```python
from build123d import *

# Parameters (mm, degrees)
SKETCH1_R               = 2.75
BOSS_EXTRUDE1_DEPTH     = 4
FILLET1_R               = 5
BOSS_EXTRUDE3_DEPTH     = 9.6
BOSS_EXTRUDE4_DEPTH     = 10
BOSS_EXTRUDE5_DEPTH     = 4
BOSS_EXTRUDE6_START     = -12
BOSS_EXTRUDE6_DEPTH     = 12
CUT_EXTRUDE1_START      = -10
CUT_EXTRUDE1_DEPTH      = 10
BOSS_EXTRUDE7_DEPTH     = 4
BOSS_EXTRUDE8_START     = -7.6
BOSS_EXTRUDE8_DEPTH     = 7.6
BOSS_EXTRUDE9_START     = 2
BOSS_EXTRUDE9_DEPTH     = 2
FILLET2_R               = 7
SKETCH15_W              = 8.45
SKETCH15_H              = 80
CUT_EXTRUDE2_DEPTH      = 14
FILLET3_R               = 2
CUT_EXTRUDE4_DEPTH      = 132.997651535
CUT_EXTRUDE4_DEPTH_BACK = 132.997651535
SKETCH17_R              = 2.75


with BuildPart() as part:
    # Sketch1 → Boss-Extrude1 (new body)
    with BuildSketch(Plane.XY):
        Polygon((-62.15, 75), (-69.55, 75), (-69.55, 65.75), (-62.15, 65.75), (-62.15, 64.25), (-69.55, 64.25), (-69.55, 55), (-62.15, 55), (-62.15, 11.5), (-41.85, 11.5), (-41.85, 55), (-34.45, 55), (-34.45, 64.25), (-41.85, 64.25), (-41.85, 65.75), (-34.45, 65.75), (-34.45, 75), (-41.85, 75), (-41.85, 118.5), (-62.15, 118.5), align=None)
        with Locations((-52, 111.75)):
            Circle(SKETCH1_R, mode=Mode.SUBTRACT)
        with Locations((-52, 18.25)):
            Circle(SKETCH1_R, mode=Mode.SUBTRACT)
    extrude(amount=BOSS_EXTRUDE1_DEPTH)

    # Fillet1
    fillet1_edges = [part.edges().sort_by_distance(p)[0] for p in [
        (-62.15, 118.5, 2),
        (-41.85, 118.5, 2),
        (-41.85, 11.5, 2),
        (-62.15, 11.5, 2),
    ]]
    fillet(fillet1_edges, radius=FILLET1_R)



with BuildPart() as body_2:
    # Sketch3 → Boss-Extrude3 (new body)
    with BuildSketch(Plane(origin=(-34.45, 0, 0), x_dir=(0, 0, -1), z_dir=(1, 0, 0))):
        with BuildLine():
            Line((-12.8, 65), (-4, 65))
            Line((-4, 65), (-4, 65.75))
            Line((-4, 65.75), (-4, 75))
            Line((-4, 75), (-4, 98.135455405))
            ThreePointArc((-4, 98.135455405), (-8.435930345, 85.488200598), (-19.8, 78.382677882))
            Line((-19.8, 78.382677882), (-19.8, 75.382677882))
            ThreePointArc((-19.8, 75.382677882), (-14.713450587, 71.260990337), (-12.8, 65))
        make_face()
        with BuildLine():
            Line((-4, 31.864544449), (-4, 65))
            Line((-4, 65), (-12.8, 65))
            ThreePointArc((-12.8, 65), (-14.713450587, 58.739009663), (-19.8, 54.617322118))
            Line((-19.8, 54.617322118), (-19.8, 51.617322118))
            ThreePointArc((-19.8, 51.617322118), (-8.435930299, 44.511799345), (-4, 31.864544449))
        make_face()
    extrude(amount=BOSS_EXTRUDE3_DEPTH)


with BuildPart() as part_1:
    add(part.part)

    add(body_2.part)  # Boss-Extrude4 merges body 2
    # Sketch5 → Boss-Extrude4 (add)
    with BuildSketch(Plane.ZY.offset(34.45)):
        with BuildLine():
            Line((4, 98.135455551), (4, 31.864544449))
            ThreePointArc((4, 31.864544449), (8.435930299, 44.511799345), (19.8, 51.617322118))
            Line((19.8, 51.617322118), (19.8, 54.617322118))
            ThreePointArc((19.8, 54.617322118), (12.8, 65), (19.8, 75.382677882))
            Line((19.8, 75.382677882), (19.8, 78.382677882))
            ThreePointArc((19.8, 78.382677882), (8.435930299, 85.488200655), (4, 98.135455551))
        make_face()
    extrude(amount=BOSS_EXTRUDE4_DEPTH)

    # Sketch6 → Boss-Extrude5 (add)
    with BuildSketch(Plane(origin=(0, 0, 4), x_dir=(-1, 0, 0), z_dir=(0, 0, -1))):
        Polygon((24.85, 31.864544449), (41.85, 31.864544449), (41.85, 55), (34.45, 55), (34.45, 64.25), (41.85, 64.25), (41.85, 65.75), (34.45, 65.75), (34.45, 75), (41.85, 75), (41.85, 98.135455551), (24.85, 98.135455551), align=None)
    extrude(amount=BOSS_EXTRUDE5_DEPTH)

    # Sketch9 → Boss-Extrude6 (add)
    with BuildSketch(Plane.ZY.offset(44.45).offset(BOSS_EXTRUDE6_START)):
        with BuildLine():
            Line((4, 31.864544449), (5, 31.864544449))
            ThreePointArc((5, 31.864544449), (9.468774813, 44.195523989), (20.8, 50.800547872))
            Line((20.8, 50.800547872), (20.8, 55.31495999))
            ThreePointArc((20.8, 55.31495999), (20.485627959, 55.424552796), (20.175, 55.544346929))
            ThreePointArc((20.175, 55.544346929), (13.8, 65), (20.175, 74.455653071))
            ThreePointArc((20.175, 74.455653071), (20.485627959, 74.575447204), (20.8, 74.68504001))
            Line((20.8, 74.68504001), (20.8, 79.199452128))
            ThreePointArc((20.8, 79.199452128), (9.468774813, 85.804476011), (5, 98.135455551))
            Line((5, 98.135455551), (4, 98.135455551))
            ThreePointArc((4, 98.135455551), (8.435930299, 85.488200655), (19.8, 78.382677882))
            Line((19.8, 78.382677882), (19.8, 75.382677882))
            ThreePointArc((19.8, 75.382677882), (12.8, 65), (19.8, 54.617322118))
            Line((19.8, 54.617322118), (19.8, 51.617322118))
            ThreePointArc((19.8, 51.617322118), (8.435930299, 44.511799345), (4, 31.864544449))
        make_face()
    extrude(amount=BOSS_EXTRUDE6_DEPTH)

    # Sketch10 → Cut-Extrude1 (cut)
    with BuildSketch(Plane.ZY.offset(44.45).offset(CUT_EXTRUDE1_START)):
        with BuildLine():
            Line((4, 98.135455551), (4, 31.864544449))
            Line((4, 31.864544449), (5, 31.864544449))
            ThreePointArc((5, 31.864544449), (9.468774813, 44.195523989), (20.8, 50.800547872))
            Line((20.8, 50.800547872), (20.8, 55.31495999))
            ThreePointArc((20.8, 55.31495999), (13.8, 65), (20.8, 74.68504001))
            Line((20.8, 74.68504001), (20.8, 79.199452128))
            ThreePointArc((20.8, 79.199452128), (9.468774813, 85.804476011), (5, 98.135455551))
            Line((5, 98.135455551), (4, 98.135455551))
        make_face()
    extrude(amount=CUT_EXTRUDE1_DEPTH, mode=Mode.SUBTRACT)

    # Sketch12 → Boss-Extrude7 (add)
    with BuildSketch(Plane.XY.offset(4)):
        Polygon((-79.15, 31.864544449), (-62.15, 31.864544449), (-62.15, 55), (-69.55, 55), (-69.55, 64.25), (-62.15, 64.25), (-62.15, 65.75), (-69.55, 65.75), (-69.55, 75), (-62.15, 75), (-62.15, 98.135455551), (-79.15, 98.135455551), align=None)
    extrude(amount=-BOSS_EXTRUDE7_DEPTH)

    # Sketch13 → Boss-Extrude8 (add)
    with BuildSketch(Plane.ZY.offset(79.15).offset(BOSS_EXTRUDE8_START)):
        with BuildLine():
            Line((19.8, 75.382677882), (19.8, 78.382677882))
            ThreePointArc((19.8, 78.382677882), (8.435930299, 85.488200655), (4, 98.135455551))
            Line((4, 98.135455551), (0, 98.135455551))
            Line((0, 98.135455551), (0, 31.864544449))
            Line((0, 31.864544449), (4, 31.864544449))
            ThreePointArc((4, 31.864544449), (8.435930299, 44.511799345), (19.8, 51.617322118))
            Line((19.8, 51.617322118), (19.8, 54.617322118))
            ThreePointArc((19.8, 54.617322118), (12.8, 65), (19.8, 75.382677882))
        make_face()
    extrude(amount=BOSS_EXTRUDE8_DEPTH)

    # Sketch14 → Boss-Extrude9 (add)
    with BuildSketch(Plane(origin=(-71.55, 0, 0), x_dir=(0, 0, -1), z_dir=(1, 0, 0)).offset(BOSS_EXTRUDE9_START)):
        with BuildLine():
            Line((-4, 98.135455551), (-5, 98.135455551))
            ThreePointArc((-5, 98.135455551), (-9.468774813, 85.804476011), (-20.8, 79.199452128))
            Line((-20.8, 79.199452128), (-20.8, 74.68504001))
            ThreePointArc((-20.8, 74.68504001), (-13.8, 65), (-20.8, 55.31495999))
            Line((-20.8, 55.31495999), (-20.8, 50.800547872))
            ThreePointArc((-20.8, 50.800547872), (-9.468774813, 44.195523989), (-5, 31.864544449))
            Line((-5, 31.864544449), (-4, 31.864544449))
            Line((-4, 31.864544449), (-4, 98.135455551))
        make_face()
    extrude(amount=-BOSS_EXTRUDE9_DEPTH)

    # Fillet2
    fillet2_edges = [part_1.edges().sort_by_distance(p)[0] for p in [
        (-24.85, 98.135455551, 2),
        (-24.85, 31.864544449, 2),
        (-41.85, 31.864544449, 2),
        (-41.85, 98.135455551, 2),
        (-79.15, 31.864544449, 2),
        (-79.15, 98.135455551, 2),
        (-62.15, 98.135455551, 2),
        (-62.15, 31.864544449, 2),
    ]]
    fillet(fillet2_edges, radius=FILLET2_R)

    # Sketch15 → Cut-Extrude2 (cut)
    with BuildSketch(Plane(origin=(0, 0, 0), x_dir=(-1, 0, 0), z_dir=(0, 0, -1))):
        with Locations((52, 65)):
            Rectangle(SKETCH15_W, SKETCH15_H)
    extrude(amount=-CUT_EXTRUDE2_DEPTH, mode=Mode.SUBTRACT)

    # Fillet3
    fillet3_edges = [part_1.edges().sort_by_distance(p)[0] for p in [
        (-28.65, 75.382677882, 19.8),
        (-28.65, 78.382677882, 19.8),
        (-28.65, 54.617322118, 19.8),
        (-28.65, 51.617322118, 19.8),
        (-33.45, 50.800547872, 20.8),
        (-33.45, 79.199452128, 20.8),
        (-33.45, 74.68504001, 20.8),
        (-33.45, 55.31495999, 20.8),
        (-75.35, 78.382677882, 19.8),
        (-75.35, 75.382677882, 19.8),
        (-75.35, 54.617322118, 19.8),
        (-75.35, 51.617322118, 19.8),
        (-70.55, 79.199452128, 20.8),
        (-70.55, 74.68504001, 20.8),
        (-70.55, 55.31495999, 20.8),
        (-70.55, 50.800547872, 20.8),
    ]]
    fillet(fillet3_edges, radius=FILLET3_R)

    # Sketch17 → Cut-Extrude4 (cut, two sides: drawn at the far end of the back side and taken through both)
    with BuildSketch(Plane(origin=(-24.85, 0, 0), x_dir=(0, 0, -1), z_dir=(1, 0, 0)).offset(-CUT_EXTRUDE4_DEPTH_BACK)):
        with Locations((-8.8, 75)):
            Circle(SKETCH17_R)
        with Locations((-8.8, 55)):
            Circle(SKETCH17_R)
    extrude(amount=CUT_EXTRUDE4_DEPTH + CUT_EXTRUDE4_DEPTH_BACK, mode=Mode.SUBTRACT)


solid = part_1.part
```
Model file for the job. Use its own axes, mm. A direction names the side the tool comes from. Coordinates: 2 decimals unless noted, no trailing zeros. Write each loop counter-clockwise with the first axis right and the second up, starting at its lowest first coordinate (ties: lowest second). Pieces come first, ordered by that corner, then holes. Notation, with made-up numbers: (28.5, 5.5) - (32.5, 5.5) arc R28 ccw to (32.5, 35.5) - close; hole circle Ø2 at (32, -11.5). An arc over 180 degrees is marked (long way). Use a Markdown table: item, result. Add a question column.
Item 1: Drop flat-ended pins along their axis: pin 1 (3.5 mm diameter, centred on x = -70.5, z = 2.5, fed in from -Y); pin 2 (3.5 mm diameter, centred on x = -70, z = 2, fed in from +Y); pin 3 (7 mm diameter, centred on x = -52, y = 18.25, fed in from +Z); pin 4 (3.5 mm diameter, centred on y = 75, z = 8.8, fed in from -X). Give the stop position or say it passes through.
Item 2: 3-axis set-ups, long thin cutter, end or side, ignore diameter. For faces 4 (the face through (-28.703, 86.216, 7.88)), 5 (the face through (-44, 66, 4)), 6 (the face through (-75.297, 43.784, 7.88)): which of +Z, -Z, +X, -X, +Y, -Y reach the whole face in a straight line?
Item 3: Band-saw the part on C-C, the plane x = -52. Write the cut outline in (y, z), and give its area (3 significant figures).
Item 4: Band-saw the part on A-A, the plane z = 2. Give the number of separate pieces and of enclosed holes in the cut face, and give its area (3 significant figures).
Item 5: Band-saw the part on B-B, the plane y = 111.75. Write the cut outline in (x, z), and give its area (3 significant figures).
Item 6: Drill centre lines: line 1 along X through (y, z) = (54, 2.25) (3 decimals); line 2 along X through (y, z) = (66.5, 7.5); line 3 along Y through (x, z) = (-53, 2). Where is each one in solid material? Low to high.
Item 7: Two-plate mould, pull along X, no slides. Class faces 1 (the face through (-56.225, 64, 2)), 2 (the face through (-62.15, 21, 2)), 3 (the face through (-75.3, 64.8, 12.8)): pulls with the +X half, pulls with the -X half, needs draft (parallel to the pull), parting line crosses it, or undercut.
A:
| question | item | result |
|---|---|---|
| 1 | pin 1 | stops at y = 31.85 |
| 1 | pin 2 | stops at y = 98.19 |
| 1 | pin 3 | stops at z = 4 |
| 1 | pin 4 | passes through |
| 2 | face 4 | +Z, +X, +Y |
| 2 | face 5 | +Z, +Y, -Y |
| 2 | face 6 | +Z, -X, -Y |
| 3 | outline | (11.5, 0) - (15.5, 0) - (15.5, 4) - (11.5, 4) - close; (21, 0) - (25, 0) - (25, 4) - (21, 4) - close; (105, 0) - (109, 0) - (109, 4) - (105, 4) - close; (114.5, 0) - (118.5, 0) - (118.5, 4) - (114.5, 4) - close |
| 3 | area | 64.0 mm² |
| 4 | separate pieces | 1 |
| 4 | enclosed holes | 3 |
| 4 | area | 3,680 mm² |
| 5 | outline | (-62.15, 0) - (-54.75, 0) - (-54.75, 4) - (-62.15, 4) - close; (-49.25, 0) - (-41.85, 0) - (-41.85, 4) - (-49.25, 4) - close |
| 5 | area | 59.2 mm² |
| 6 | line 1 | x = -79.15 to -56.225, -47.775 to -24.85 |
| 6 | line 2 | x = -79.15 to -69.55, -34.45 to -24.85 |
| 6 | line 3 | y = 11.5 to 15.69, 20.81 to 25, 105 to 109.19, 114.31 to 118.5 |
| 7 | face 1 | undercut |
| 7 | face 2 | pulls with the -X half |
| 7 | face 3 | needs draft |
